Source: CAD feature listing. Evaluate the final solid. Frame: model axes, mm. Face numbers are marked on the shaded views. A direction names the side the tool comes from. Coordinates: 2 decimals unless noted, no trailing zeros. Write each loop counter-clockwise with the first axis right and the second up, starting at its lowest first coordinate (ties: lowest second). Pieces come first, ordered by that corner, then holes. Notation, with made-up numbers: (-7, 15) -> (39, 15) arc R14 cw to (39, 42) -> close; hole circle Ø4 at (65, 10). An arc over 180 degrees is marked (long way). One line per item, written item: value. Start each with the question number.
1. Section query A-A, the plane z = -19. Output: boundary loops of the cut face in (x, y), and give its area (3 significant figures).
2. Line query: line 1 (X direction, y = -3.75, z = -5); line 2 (Z direction, x = 7.5, y = -3.85); line 3 (Z direction, x = 7.5, y = -3.35). Output: solid intervals per line, ascending.
3. Section query C-C, the plane x = 6.5. Output: boundary loops of the cut face in (y, z), and give its area (3 significant figures).
4. Section query D-D, the plane z = 8.5. Output: boundary loops of the cut face in (x, y), and give its area (3 significant figures).
5. First-contact query: P1, Ø3, axis at x = 7.5, z = 8.5, coming from the -Y side; P2, Ø2.5, axis at x = 9.5, y = 4.5, coming from the -Z side; P3, Ø3, axis at x = -5.5, z = 3, coming from the -Y side; P4, Ø1.5, axis at x = -2, y = -14.5, coming from the -Z side. Flat tips, straight axial feed; report the tip coordinate or a pass-through.
6. Section query B-B, the plane y = 4. Output: boundary loops of the cut face in (x, z).
7. Mould query, pull axis Z, two halves, no side actions, for the marked faces 1, 2, 3 and 4. Classes: released by +Z, released by -Z, zero draft, split by the parting line, or undercut.
8. Access query for the marked faces 5, 6, 7 and 8. Directions: +Z, -Z, +X, -X, +Y, -Y. A direction counts if a zero-diameter tool reaches every point of the face in a straight line with its end or side. Return the directions, or none.
Autodesk Inventor part; units mm, degrees
ref_plane "YZ Plane" through (0, 0, 0) normal (1, 0, 0) x (0, 1, 0)
ref_plane "XZ Plane" through (0, 0, 0) normal (0, 1, 0) x (-1, 0, 0)
ref_plane "XY Plane" through (0, 0, 0) normal (0, 0, 1) x (1, 0, 0)
sketch "Sketch1" plane through (0, 0, 0) normal (0, 1, 0) x (-1, 0, 0)
  line L0 (15, 13.5) -> (15, -13.5)
  line L1 (15, -13.5) -> (-15, -13.5)
  line L2 (-15, -13.5) -> (-15, 13.5)
  line L3 (-15, 13.5) -> (15, 13.5)
  point P0 (0, -13.5)
  point P1 (-15, 0)
  dimension "d2" = 27
  dimension "d3" = 30
extrude "Extrusion1" [suppressed]
sketch "Sketch4" plane through (0, 0, 0) normal (1, 0, 0) x (0, 1, 0)
  line L0 (-18.1177, -21.5508) -> (-25.8677, 7.3726)
  line L1 (0, 13.5) -> (-3, 13.5)
  line L2 (-17.057, -19.7137) -> (-4.5, -16.349)
  line L3 (-4.5, 11.5452) -> (-24.0306, 6.312)
  line L4 (-3, -17.5) -> (-3, 13.5)
  line L5 (-24.0306, 6.312) -> (-17.057, -19.7137)
  line L6 (-4.5, -16.349) -> (-4.5, 11.5452)
  line L7 (-3, -13.5) -> (-3, 13.5)
  line L8 (-3, 13.5) -> (-25.8677, 7.3726)
  line L9 (-3, -17.5) -> (-18.1177, -21.5508)
  point P0 (0, 0)
  point P1 (-51.8403, 80.9842)
  point P2 (-3, 0)
  point P3 (-3, 0)
  point P4 (-3, 0)
  point P5 (-14.2653, 8.9286)
  point P6 (-10.5588, -19.5254)
  dimension "d50" = 1.5
  dimension "d57" = 1.5
  dimension "d59" = 1.5
  dimension "d60" = 1.5
  dimension "d62" = 4
  dimension "d63" = 15
  dimension "d64" = 13
extrude "Extrusion3" add sketch "Sketch4" along normal mid plane 22
sketch "Sketch5" plane through (11, 0, 0) normal (1, 0, 0) x (0, 0, -1)
  line L0 (17.5, -3) -> (-13.5, -3)
  line L1 (14.5, -3) -> (17.5, -3)
  line L2 (17.5, -3) -> (17.5, 7)
  line L3 (17.5, 7) -> (14.5, 7)
  line L4 (14.5, 7) -> (14.5, -3)
  point P0 (0, 0)
  point P1 (13.5, -3)
  dimension "d67" = 3
  dimension "d68" = 10
extrude "Extrusion4" add sketch "Sketch5" against normal blind 5
mirror "Mirror1" about plane through (0, 0, 0) normal (1, 0, 0) of "Extrusion4"
sketch "Sketch6" plane through (0, -3, 0) normal (0, 1, 0) x (1, 0, 0)
  line L0 (15, 13.5) -> (15, -13.5)
  line L1 (11, -13.5) -> (-11, -13.5)
  line L2 (-11, 13.5) -> (11, 13.5)
  point P0 (0, 0)
  point P1 (-7.5, 5)
  point P2 (7.5, 5)
  point P3 (7.5, -8.5)
  point P4 (-7.5, -8.5)
  dimension "d71" = 15
  dimension "d72" = 13.5
  dimension "d73" = 7.5
  dimension "d74" = 5
  dimension "d75" = 8.5
hole "Hole2" at (-7.5, -3, -5) at (7.5, -3, -5) at (7.5, -3, 8.5) at (-7.5, -3, 8.5) direction (0, -1, 0) diameter 3.4 depth 1.5
sketch "Sketch7" plane through (-11, -24.0306, 6.312) normal (0, 0.9659258, 0.258819) x (1, 0, 0)
  line L0 (22, -1.5) -> (0, -1.5)
  line L1 (22, -1.5) -> (22, 28.4437)
  point P0 (11, 12.3165)
  point P1 (3.5, 19)
  point P2 (18.5, 19)
  point P3 (18.5, 5.5)
  point P4 (3.5, 5.5)
  dimension "d83" = 15
  dimension "d84" = 13.5
  dimension "d88" = 7
  dimension "d89" = 3.5
hole "Hole3" at (-7.5, -22.6071, 0.9994) at (7.5, -22.6071, 0.9994) at (7.5, -19.113, -12.0406) at (-7.5, -19.113, -12.0406) direction (0, -0.9659258, -0.258819) diameter 3.4 depth 1.5
properties part number "Ramp"
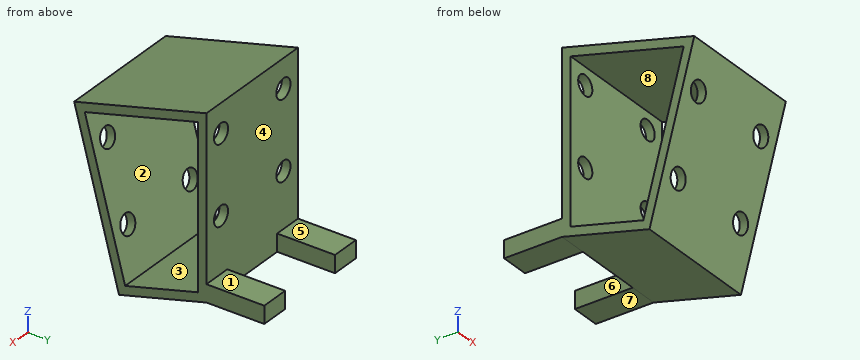
Computed values:
1. outline: (-11, -18.8) -> (11, -18.8) -> (11, -17.25) -> (-11, -17.25) -> close; (-11, -14.39) -> (11, -14.39) -> (11, -8.6) -> (-11, -8.6) -> close
1. area: 162 mm²
2. line 1: x = -11 to -9.2, -5.8 to 5.8, 9.2 to 11
2. line 2: z = -17.73 to -6.7, -3.3 to 6.8, 10.2 to 13.27
2. line 3: z = -17.59 to -6.7, -3.3 to 6.8, 10.2 to 13.41
3. outline: (-25.87, 7.37) -> (-24.41, 1.94) -> (-22.96, 2.33) -> (-24.03, 6.31) -> (-4.5, 11.55) -> (-4.5, 9.87) -> (-3, 9.87) -> (-3, 13.5) -> close; (-23.7, -0.72) -> (-20.92, -11.1) -> (-19.47, -10.71) -> (-22.25, -0.33) -> close; (-20.21, -13.76) -> (-18.12, -21.55) -> (-3, -17.5) -> (7, -17.5) -> (7, -14.5) -> (-3, -14.5) -> (-3, -6.37) -> (-4.5, -6.37) -> (-4.5, -16.35) -> (-17.06, -19.71) -> (-18.76, -13.37) -> close; (-4.5, -3.63) -> (-3, -3.63) -> (-3, 7.13) -> (-4.5, 7.13) -> close
3. area: 155 mm²
4. outline: (-11, -21.66) -> (11, -21.66) -> (11, -15.86) -> (-11, -15.86) -> close; (-11, -4.5) -> (-9.2, -4.5) -> (-9.2, -3) -> (-11, -3) -> close; (-5.8, -4.5) -> (5.8, -4.5) -> (5.8, -3) -> (-5.8, -3) -> close; (9.2, -4.5) -> (11, -4.5) -> (11, -3) -> (9.2, -3) -> close
4. area: 150 mm²
5. P1: stops at y = -25.87
5. P2: stops at z = -17.5
5. P3: stops at y = -25.1
5. P4: stops at z = -20.78
6. outline: (-11, -17.5) -> (-6, -17.5) -> (-6, -14.5) -> (-11, -14.5) -> close; (6, -17.5) -> (11, -17.5) -> (11, -14.5) -> (6, -14.5) -> close
7. face 1: released by +Z
7. face 2: undercut
7. face 3: undercut
7. face 4: zero draft
8. face 5: +Z, +X, -X, +Y
8. face 6: +Z, -Z, +Y
8. face 7: -Z, +X, -X, +Y
8. face 8: +X, -X
